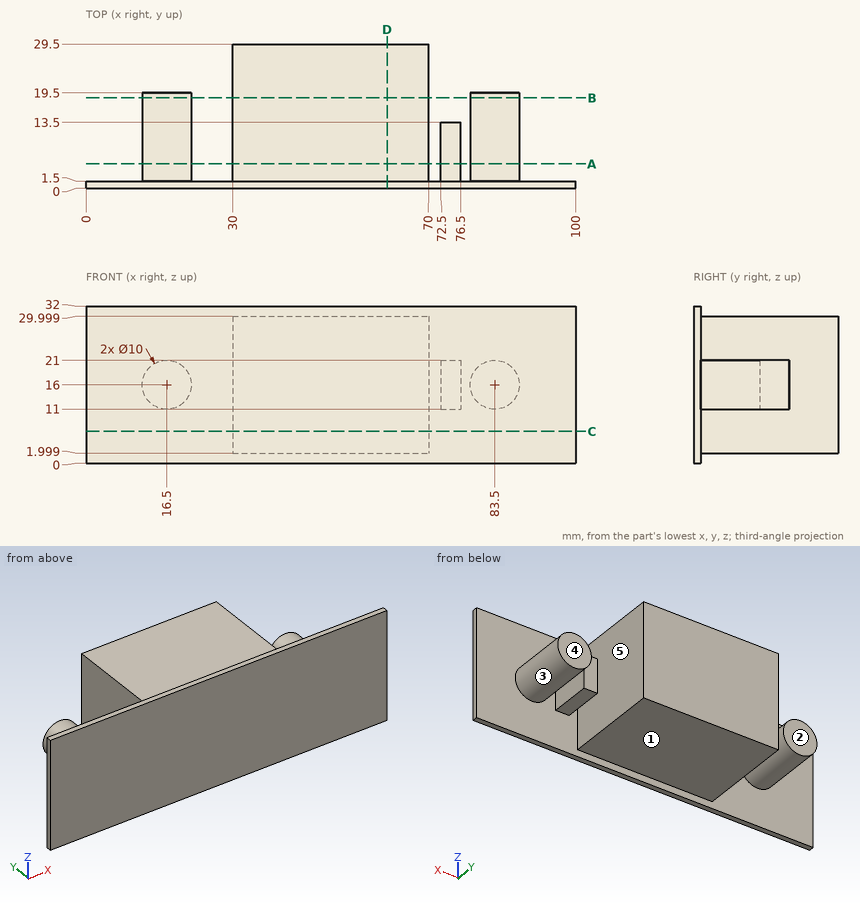
Could you check a few things on this drawing? It's one solid part, dimensions in mm from its lowest x, y, z. A direction names the side the tool comes from. Give positions to 0.01 mm unless a question says otherwise; leave off trailing zeros. Loops run counter-clockwise (first coordinate to the right, second up) from the corner with the lowest first, then second, coordinate; pieces in that order, holes last. Notation, with made-up numbers: M 78.25,56 L 116.25,56 A20 cw 116.25,74 Z; hole C -31,-34 d4. An arc over 180 degrees is marked long. Return JSON: item names as keys, results as strings.
Item 1: Please list where these lines run through material, in increasing order: line 1 (Y direction, x = 10, z = 25); line 2 (X direction, y = 14, z = 24.5); line 3 (X direction, y = 4, z = 19.5).
A:
{"line 1": "y = 0 to 1.5", "line 2": "x = 30 to 70", "line 3": "x = 12.93 to 20.07, 30 to 70, 72.5 to 76.5, 79.93 to 87.07"}
Item 2: I'm going to push flat-ended pins straight in: pin 1 Ø14 at (y, z) = (11, 17.5) entering from -X; pin 2 Ø5 at (y, z) = (5.5, 16.5) entering from +X; pin 3 Ø5 at (x, z) = (83.5, 15) entering from +Y. Where does each tip first touch, or does it pass through?
A:
{"pin 1": "stops at x = 11.5", "pin 2": "stops at x = 88.5", "pin 3": "stops at y = 19.5"}
Item 3: Thinking about a two-plate mould opening in X: for the marked faces 4 and 5, which applies, released by +X, released by -X, zero draft, split by the parting line, or undercut?
A:
{"face 4": "zero draft", "face 5": "undercut"}
Item 4: Imagine slicing it at D-D on x = 61.5. List the corners of the cut face in (y, z) for me, then the cut area to 3 significant figures.
A:
{"outline": "M 0,0 L 1.5,0 L 1.5,2 L 29.5,2 L 29.5,30 L 1.5,30 L 1.5,32 L 0,32 Z", "area": "832 mm^2"}
Item 5: On a 3-axis mill with a long thin cutter (end or side, diameter ignored), from which of +Z, -Z, +X, -X, +Y, -Y can I reach the whole of each face in a straight line? I mean the marked faces 1, 2 and 3. Say none if no direction works.
A:
{"face 1": "-Z, +X, -X, +Y", "face 2": "+Z, -Z, -X, +Y", "face 3": "+Y"}
Item 6: Imagine slicing it at A-A on y = 5. List the corners of the cut face in (x, z) for me.
A:
{"outline": "C 16.5,16 d10; M 30,2 L 70,2 L 70,30 L 30,30 Z; M 72.5,11 L 76.5,11 L 76.5,21 L 72.5,21 Z; C 83.5,16 d10"}
Item 7: Imagine slicing it at B-B on y = 18.5. List the corners of the cut face in (x, z) for me, then the cut area to 3 significant figures.
A:
{"outline": "C 16.5,16 d10; M 30,2 L 70,2 L 70,30 L 30,30 Z; C 83.5,16 d10", "area": "1,280 mm^2"}
Item 8: Imagine slicing it at C-C on z = 6.5. List the corners of the cut face in (x, y) for me, then the cut area to 3 significant figures.
A:
{"outline": "M 0,0 L 100,0 L 100,1.5 L 70,1.5 L 70,29.5 L 30,29.5 L 30,1.5 L 0,1.5 Z", "area": "1,270 mm^2"}
